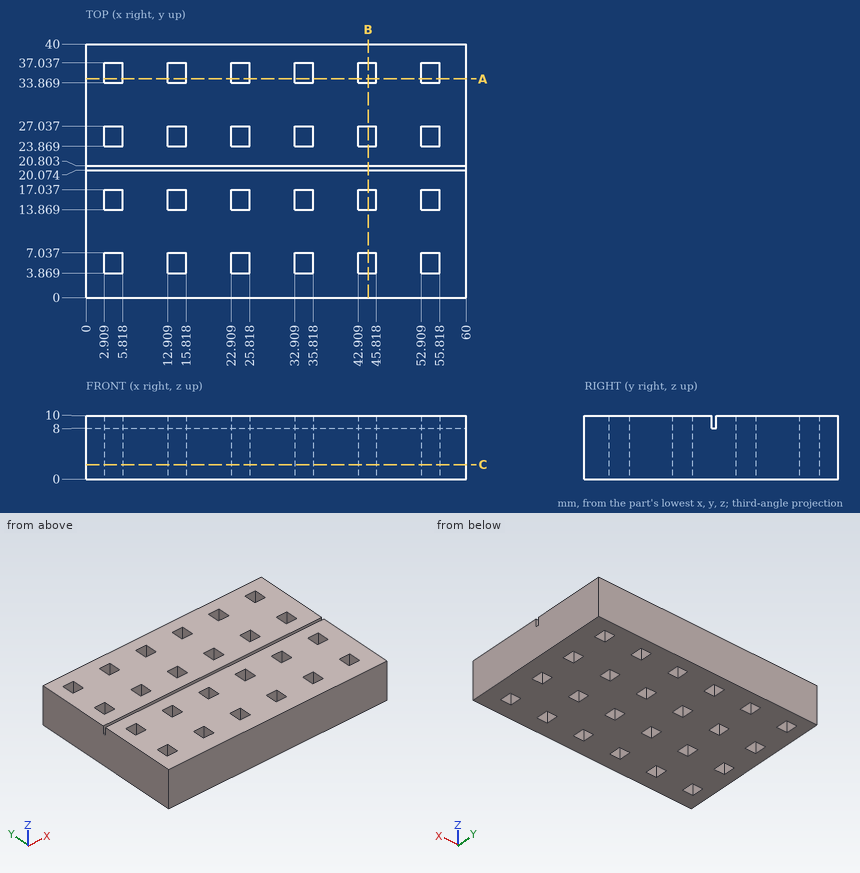
Design review of the part shown in the three views and the two pictorial views. Dimensions are in mm from the part's minimum x, y and z. Round coordinates to 2 decimals unless told otherwise and drop trailing zeros. Loops run counter-clockwise (first coordinate to the right, second up) from the corner with the lowest first, then second, coordinate; pieces in that order, holes last. Notation, with made-up numbers: (30, 83) -> (70, 83) arc R21 ccw to (70, 104) -> close; hole circle Ø3 at (30, 61.5). An arc over 180 degrees is marked (long way). Use one line per item in the form item = value. Start each with the question number.
Q1. We need section A-A on y = 34.5. Give the boundary of the cut face in (x, z).
Q2. We need section B-B on x = 44.5. Give the boundary of the cut face in (y, z).
Q3. We need section C-C on z = 2.25. State how many separate pieces and enclosed holes the cut face has, then the cut area to 3 significant figures.
Q4. Wall thickness on line 1 along Y through (x, z) = (43, 9); line 2 along Y through (x, z) = (14, 7.25); line 3 along Y through (x, z) = (27.5, 8.5): over which ranges is each line inside the solid? List them lowest first. Write a range as [from, to].
Calculated:
q1.outline = (0, 0) -> (2.91, 0) -> (2.91, 10) -> (0, 10) -> close; (5.82, 0) -> (12.91, 0) -> (12.91, 10) -> (5.82, 10) -> close; (15.82, 0) -> (22.91, 0) -> (22.91, 10) -> (15.82, 10) -> close; (25.82, 0) -> (32.91, 0) -> (32.91, 10) -> (25.82, 10) -> close; (35.82, 0) -> (42.91, 0) -> (42.91, 10) -> (35.82, 10) -> close; (45.82, 0) -> (52.91, 0) -> (52.91, 10) -> (45.82, 10) -> close; (55.82, 0) -> (60, 0) -> (60, 10) -> (55.82, 10) -> close
q2.outline = (0, 0) -> (3.87, 0) -> (3.87, 10) -> (0, 10) -> close; (7.04, 0) -> (13.87, 0) -> (13.87, 10) -> (7.04, 10) -> close; (17.04, 0) -> (23.87, 0) -> (23.87, 10) -> (20.8, 10) -> (20.8, 8) -> (20.07, 8) -> (20.07, 10) -> (17.04, 10) -> close; (27.04, 0) -> (33.87, 0) -> (33.87, 10) -> (27.04, 10) -> close; (37.04, 0) -> (40, 0) -> (40, 10) -> (37.04, 10) -> close
q3.separate_pieces = 1
q3.enclosed_holes = 24
q3.area = 2,180 mm²
q4.line_1 = [0, 3.87], [7.04, 13.87], [17.04, 20.07], [20.8, 23.87], [27.04, 33.87], [37.04, 40]
q4.line_2 = [0, 3.87], [7.04, 13.87], [17.04, 23.87], [27.04, 33.87], [37.04, 40]
q4.line_3 = [0, 20.07], [20.8, 40]
